```python
from build123d import *

# Parameters (mm, degrees)
BOSS_EXTRUDE1_DEPTH = 75
SKETCH2_R           = 5
CUT_EXTRUDE1_DEPTH  = 10
SKETCH4_R           = 2.341017376
CUT_EXTRUDE2_DEPTH  = 10


with BuildPart() as part:
    # Sketch1 → Boss-Extrude1 (new body)
    with BuildSketch(Plane.XY):
        with BuildLine():
            Line((0, 0), (0, 20))
            ThreePointArc((0, 20), (-7.495083498, 7.495083498), (-20, 0))
            Line((-20, 0), (0, 0))
        make_face()
    extrude(amount=BOSS_EXTRUDE1_DEPTH)

    # Sketch2 → Cut-Extrude1 (cut)
    with BuildSketch(Plane(origin=(0, 0, 0), x_dir=(0, 0, -1), z_dir=(1, 0, 0))):
        with Locations((-30, 21.3)):
            Circle(SKETCH2_R)
    extrude(amount=-CUT_EXTRUDE1_DEPTH, mode=Mode.SUBTRACT)

    # Sketch4 → Cut-Extrude2 (cut)
    with BuildSketch(Plane(origin=(0, 0, 0), x_dir=(-1, 0, 0), z_dir=(0, -1, 0))):
        with Locations((18.11370574, -59.963970786)):
            Circle(SKETCH4_R)
    extrude(amount=-CUT_EXTRUDE2_DEPTH, mode=Mode.SUBTRACT)


solid = part.part
```
Verification items for the finished model (mm, model axes). Coordinates: 2 decimals unless noted, no trailing zeros. Order: outer loops, then holes, each group sorted by start corner. A loop starts at its lowest first (then second) coordinate and runs counter-clockwise, first axis right, second up. Notation, with made-up numbers: (-40, 50) -> (1, 50) arc R29 cw to (1, 85) -> close; hole circle Ø3 at (-35, 32.25). An arc over 180 degrees is marked (long way). Answer as CSV lines item,"result". Start each with the question number.
1) Gauge pin test, flat ends, axial feed: pin 1 Ø8 at (x, z) = (-4, 38.5) entering from -Y; pin 2 Ø6 at (x, z) = (-18.11, 59.96) entering from +Y; pin 3 Ø3 at (y, z) = (14.5, 46) entering from -X; pin 4 Ø2 at (y, z) = (15.5, 37.5) entering from -X. Record the tip position at first contact, or that the pin passes through.
2) Cross-section at D-D, the plane x = -13.25. Record the boundary of the cut face in (y, z), then the cut area to 3 significant figures.
3) Material ranges on L1, parallel to X at y = 1.75, z = 71.5; L2, parallel to X at y = 16.5, z = 27; L3, parallel to Y at x = -2, z = 61, recorded low to high. Write a range as [from, to].
4) Cross-section at A-A, the plane x = -17.25. Record the boundary of the cut face in (y, z).
5) Cross-section at C-C, the plane z = 26. Record the boundary of the cut face in (x, y), then the cut area to 3 significant figures.
6) Release check for a two-part mould opening along Z. For faces 1 (the face through (-0.5, 16.3, 30.1)), 2 (the face through (-6, 6, 75)), 3 (the face through (-6, 6, 0)), 4 (the face through (-10, 0, 37)) record: released by +Z, released by -Z, zero draft, split by the parting line, or undercut.
7) Cross-section at B-B, the plane y = 17.5. Record the boundary of the cut face in (x, z).
Conclusion:
1,pin 1,"stops at y = 0"
1,pin 2,"stops at y = 1.97"
1,pin 3,"stops at x = -3.15"
1,pin 4,"stops at x = -2.29"
2,outline,"(0, 0) -> (3, 0) -> (3, 75) -> (0, 75) -> close"
2,area,"225 mm²"
3,L1,"x = [-15.55, 0]"
3,L2,"x = [-1.3, 0]"
3,L3,"y = [0, 15.05]"
4,outline,"(0, 0) -> (0.98, 0) -> (0.98, 57.79) -> (0, 57.79) -> close; (0, 62.14) -> (0.98, 62.14) -> (0.98, 75) -> (0, 75) -> close"
5,outline,"(-20, 0) -> (0, 0) -> (0, 18.3) -> (-0.57, 18.3) arc R30 cw to start"
5,area,"132 mm²"
6,face 1,"undercut"
6,face 2,"released by +Z"
6,face 3,"released by -Z"
6,face 4,"zero draft"
7,outline,"(-0.88, 0) -> (0, 0) -> (0, 26.75) -> (-0.88, 26.75) -> close; (-0.88, 33.25) -> (0, 33.25) -> (0, 75) -> (-0.88, 75) -> close"
